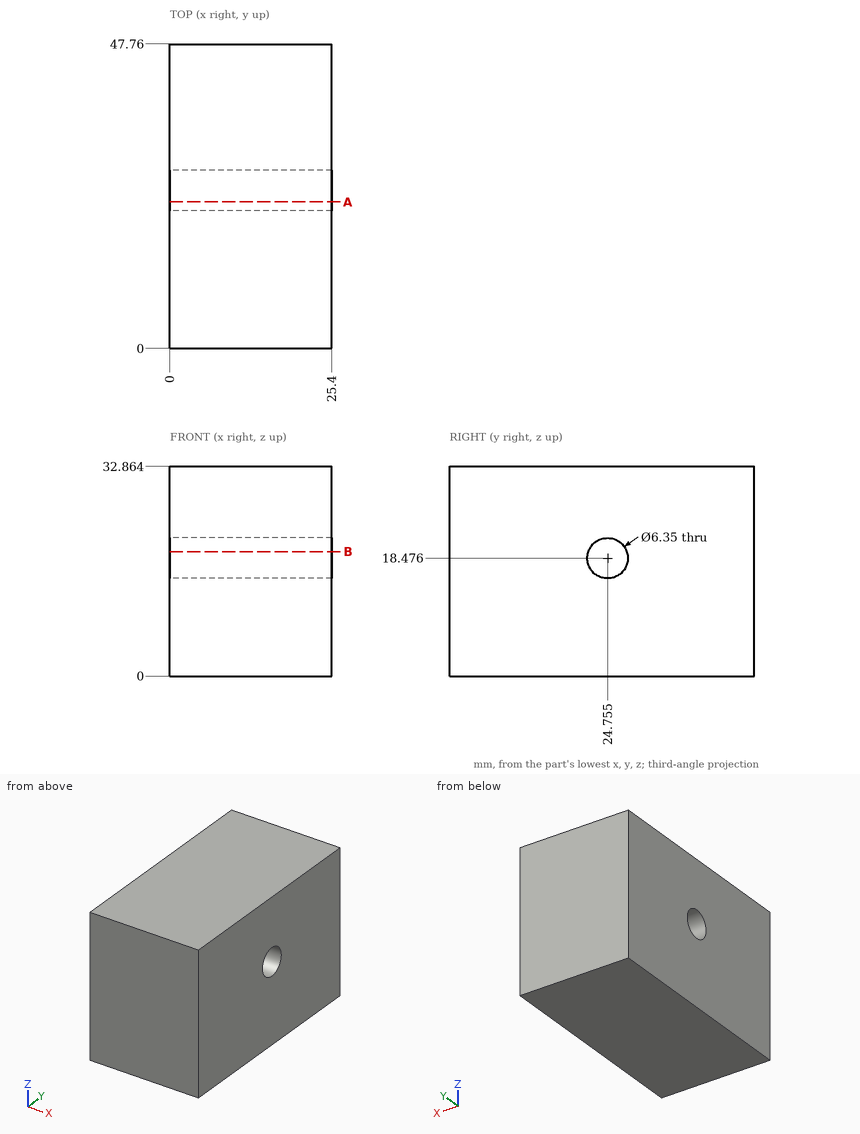
The figure shows three views and two pictorial views of one solid part (mm, origin at its lowest corner). Answer the questions. Give positions to 0.01 mm unless a question says otherwise; leave off trailing zeros. Write each loop counter-clockwise with the first axis right and the second up, starting at its lowest first coordinate (ties: lowest second). Pieces come first, ordered by that corner, then holes. Notation, with made-up numbers: M 30.25,-21.5 L 39.25,-21.5 A27 cw 39.25,1.5 Z; hole C 25,17.5 d3. An arc over 180 degrees is marked long. One line per item, written item: value. Start each with the question number.
(1) Find section B-B (z = 19.5). Determine the outline of the cut face in (x, y).
(2) Find the intervals of material crossed by line 1 (Y direction, x = 5.75, z = 17.5) (1 decimal); line 2 (Y direction, x = 16, z = 16.5); line 3 (Z direction, x = 5.75, y = 25.5), in increasing order.
(3) A flat-ended cylindrical pin translates along its axis: pin 1 Ø4 at (y, z) = (24.76, 18.48) entering from -X. Find the tip coordinate at first contact, or state that the pin passes through.
(4) Find section A-A (y = 23). Determine the outline of the cut face in (x, z).
Results below:
1. outline: M 0,0 L 25.4,0 L 25.4,21.75 L 0,21.75 Z; M 0,27.76 L 25.4,27.76 L 25.4,47.76 L 0,47.76 Z
2. line 1: y = 0 to 21.7, 27.8 to 47.8
2. line 2: y = 0 to 22.27, 27.24 to 47.76
2. line 3: z = 0 to 15.39, 21.56 to 32.86
3. pin 1: passes through
4. outline: M 0,0 L 25.4,0 L 25.4,15.83 L 0,15.83 Z; M 0,21.12 L 25.4,21.12 L 25.4,32.86 L 0,32.86 Z
